Can you work these out from the model? Positions are in its coordinate system, mm. A direction names the side the tool comes from. Coordinates: 2 decimals unless noted, no trailing zeros. Write each loop counter-clockwise with the first axis right and the second up, starting at its lowest first coordinate (ties: lowest second). Pieces come first, ordered by that corner, then holes.
```python
from build123d import *

# Parameters (mm, degrees)
F0_R     = 32
F3_DEPTH = 2
F1_R     = 28.675
F4_DEPTH = 6.5
F2_R     = 24
F5_DEPTH = 10
F6_SIZE  = 1.5
F7_R     = 1


with BuildPart() as f3:
    # F0 (on Top) → F3 (new body)
    with BuildSketch(Plane.XY):
        Circle(F0_R)
    extrude(amount=-F3_DEPTH)

    # F1 (on Top) → F4 (join)
    with BuildSketch(Plane.XY):
        Circle(F1_R)
    extrude(amount=F4_DEPTH)

    # F2 (on Top) → F5 (cut, symmetric)
    with BuildSketch(Plane.XY):
        Circle(F2_R)
    extrude(amount=F5_DEPTH, both=True, mode=Mode.SUBTRACT)

    # F6
    f6_edges = [f3.edges().sort_by_distance(p)[0] for p in [
        (-28.675, 0, 6.5),
    ]]
    chamfer(f6_edges, length=F6_SIZE)

    # F7
    f7_edges = [f3.edges().sort_by_distance(p)[0] for p in [
        (-24, 0, -2),
        (-32, 0, -2),
    ]]
    fillet(f7_edges, radius=F7_R)


solid = f3.part
```
1. I'm going to push flat-ended pins straight in: P1, Ø4, axis at y = -24, z = 4, coming from the +X side; P2, Ø1, axis at x = 11, z = 0, coming from the -Y side; P3, Ø3, axis at y = -16, z = 5, coming from the -X side. Where does each tip first touch, or does it pass through?
2. We'd pull the mould along X, two halves only. Please class faces 1 (the face through (27.35, 8.61, 2.46)), 2 (the face through (-21, 14, -2)), 3 (the face through (-23.977, 1.055, 2.802)): released by +X, released by -X, zero draft, split by the parting line, or undercut.
3. If I drill on L1, parallel to Y at x = 0, z = 2.25 (3 decimals); L2, parallel to Y at x = 22, z = -1; L3, parallel to X at y = -17.5, z = 3.25, over which ranges is the centre line in solid material (lowest first)?
4. If we section it at A-A, the plane y = 0: List the corners of the cut face in (x, z) for me (3 decimals), plus the area to 3 significant figures.
5. Which directions (+Z, -Z, +X, -X, +Y, -Y) give clear straight access to the entire face, cutting with the end or side of a thin tool? Please do faces 4 (the face through (-29, -2, 0)), 5 (the face through (-6.94, -31.24, -0.49)).
Answers:
1. P1: stops at x = 18.39
1. P2: stops at y = -30.23
1. P3: stops at x = -24.74
2. face 1: split by the parting line
2. face 2: zero draft
2. face 3: undercut
3. L1: y = -28.675 to -24, 24 to 28.675
3. L2: y = -23.24 to -9.59, 9.59 to 23.24
3. L3: x = -22.72 to -16.42, 16.42 to 22.72
4. outline: (-32, -1) arc R1 ccw to (-31, -2) - (-25, -2) arc R1 ccw to (-24, -1) - (-24, 6.5) - (-27.175, 6.5) - (-28.675, 5) - (-28.675, 0) - (-32, 0) - close; (24, -1) arc R1 ccw to (25, -2) - (31, -2) arc R1 ccw to (32, -1) - (32, 0) - (28.675, 0) - (28.675, 5) - (27.175, 6.5) - (24, 6.5) - close
4. area: 89.7 mm2
5. face 4: +Z
5. face 5: +Z, -Z
